Part print with two shaded views. Sizes in mm from the minimum x, y, z corner. Give positions to 0.01 mm unless a question says otherwise; leave off trailing zeros. Write each loop counter-clockwise with the first axis right and the second up, starting at its lowest first coordinate (ties: lowest second). Pieces come first, ordered by that corner, then holes. Notation, with made-up numbers: (-16, 32.25) -> (21, 32.25) arc R16 ccw to (21, 48.25) -> close; hole circle Ø5 at (46.25, 2). An arc over 180 degrees is marked (long way). Answer as a JSON object with one key per item and string values.
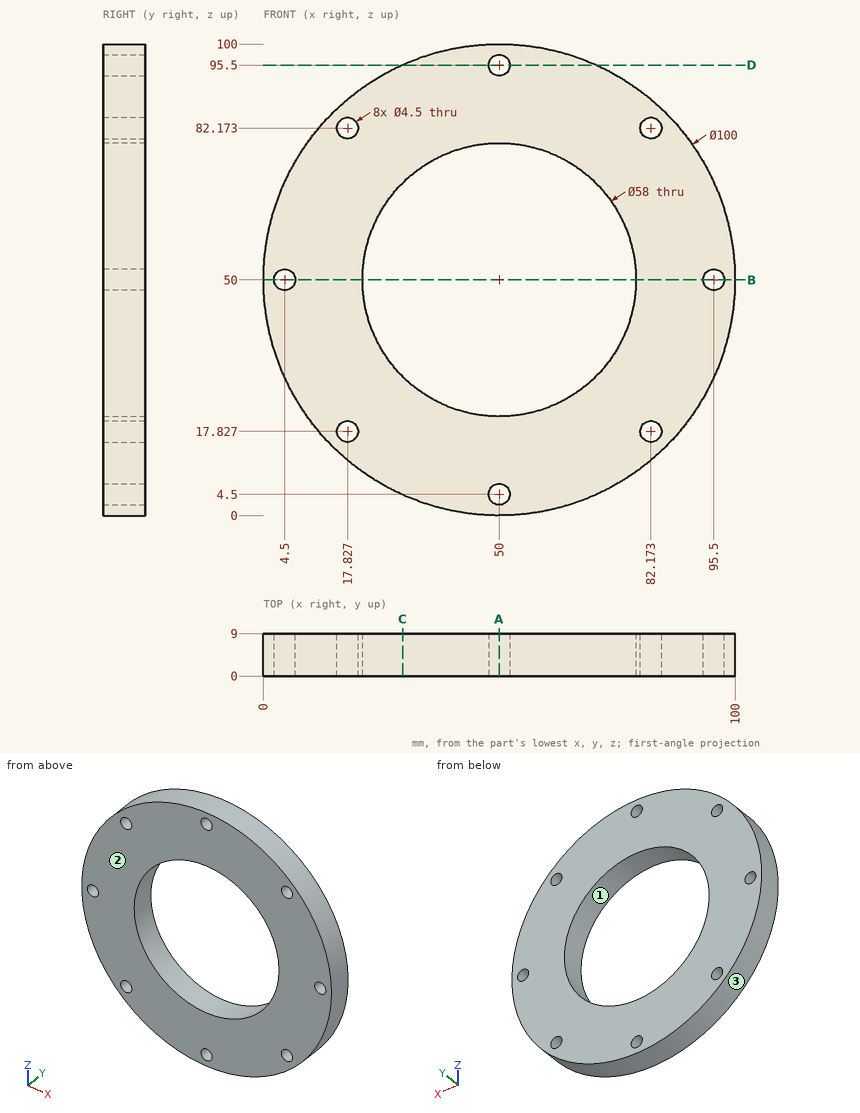
1) Pin check, flat tips, straight feed: pin 1 (4 mm diameter, centred on x = 72, y = 6, fed in from -Z) (1 decimal); pin 2 (1.5 mm diameter, centred on x = 13, y = 4.5, fed in from +Z); pin 3 (2 mm diameter, centred on y = 8, z = 39.5, fed in from -X). Stop position of each tip, or through.
Model answer:
{"pin 1": "stops at z = 4.2", "pin 2": "stops at z = 84.44", "pin 3": "stops at x = 0.91"}
2) Slice it at B-B (z = 50). List the corners of the cut face in (x, y).
Model answer:
{"outline": "(0, 0) -> (2.25, 0) -> (2.25, 9) -> (0, 9) -> close; (6.75, 0) -> (21, 0) -> (21, 9) -> (6.75, 9) -> close; (79, 0) -> (93.25, 0) -> (93.25, 9) -> (79, 9) -> close; (97.75, 0) -> (100, 0) -> (100, 9) -> (97.75, 9) -> close"}
3) Mould opens along Z. For the marked faces 1, 2 and 3 say: released by +Z, released by -Z, zero draft, split by the parting line, or undercut.
Model answer:
{"face 1": "undercut", "face 2": "zero draft", "face 3": "split by the parting line"}
4) Slice it at C-C (x = 29.5). List the corners of the cut face in (y, z) (1 decimal).
Model answer:
{"outline": "(0, 4.4) -> (9, 4.4) -> (9, 29.5) -> (0, 29.5) -> close; (0, 70.5) -> (9, 70.5) -> (9, 95.6) -> (0, 95.6) -> close"}
5) Slice it at A-A (x = 50). List the corners of the cut face in (y, z).
Model answer:
{"outline": "(0, 0) -> (9, 0) -> (9, 2.25) -> (0, 2.25) -> close; (0, 6.75) -> (9, 6.75) -> (9, 21) -> (0, 21) -> close; (0, 79) -> (9, 79) -> (9, 93.25) -> (0, 93.25) -> close; (0, 97.75) -> (9, 97.75) -> (9, 100) -> (0, 100) -> close"}
6) Slice it at D-D (z = 95.5). List the corners of the cut face in (x, y).
Model answer:
{"outline": "(29.27, 0) -> (47.75, 0) -> (47.75, 9) -> (29.27, 9) -> close; (52.25, 0) -> (70.73, 0) -> (70.73, 9) -> (52.25, 9) -> close"}
7) Wall check: probe 1 along X at (y, z) = (5, 50); probe 2 along Z at (x, y) = (83, 0.5) (1 decimal); probe 3 along X at (y, z) = (2.75, 74) (1 decimal). Give the ranges that are in metal, low to high.
Model answer:
{"probe 1": "x = 0 to 2.25, 6.75 to 21, 79 to 93.25, 97.75 to 100", "probe 2": "z = 12.4 to 15.7, 19.9 to 80.1, 84.3 to 87.6", "probe 3": "x = 6.1 to 33.7, 66.3 to 93.9"}
